from build123d import *

# Parameters (mm, degrees)
BOSS_EXTRUDE1_DEPTH       = 10
SKETCH3_W                 = 6
SKETCH3_H                 = 5
CHAMFER1_SIZE             = 4
SKETCH10_R                = 6.5
CUT_EXTRUDE1_DEPTH        = 11
F_6_0MM_DOWEL_HOLE1_D     = 6
F_6_0MM_DOWEL_HOLE1_DEPTH = 4
F_6_0MM_DOWEL_HOLE1_TIP   = 1.802581857


with BuildPart() as part:
    # Sketch1 → Boss-Extrude1 (new body)
    with BuildSketch(Plane(origin=(0, 0, 0), x_dir=(1, 0, 0), z_dir=(0, 1, 0))):
        Polygon((0, -85), (0, -50), (-50, -50), (-50, 50), (0, 50), (0, 85), (-85, 85), (-85, -85), align=None)
    extrude(amount=BOSS_EXTRUDE1_DEPTH)

    # Cut-Sweep1: sweep along a path in Sketch4
    with BuildLine(Plane.XZ) as cut_sweep1_path:
        Line((0, 50), (-50, 50))
        Line((-50, 50), (-50, -50))
        Line((-50, -50), (0, -50))
    # Sketch3 → Cut-Sweep1 (sweep, cut)
    with BuildSketch(Plane(origin=(0, 0, 0), x_dir=(0, 0, -1), z_dir=(1, 0, 0))):
        with Locations((-53, 2.5)):
            Rectangle(SKETCH3_W, SKETCH3_H)
    sweep(path=cut_sweep1_path.line, transition=Transition.RIGHT, mode=Mode.SUBTRACT)

    # Chamfer1
    chamfer1_edges = [part.edges().sort_by_distance(p)[0] for p in [
        (0, 10, 67.5),
        (0, 10, -67.5),
    ]]
    chamfer(chamfer1_edges, length=CHAMFER1_SIZE)

    # Sketch10 → Cut-Extrude1 (cut, through all)
    with BuildSketch(Plane(origin=(0, 10, 0), x_dir=(1, 0, 0), z_dir=(0, 1, 0))):
        with Locations((-72.499960031, 0)):
            Circle(SKETCH10_R)
        with Locations((-20, -72.5)):
            Circle(SKETCH10_R)
        with Locations((-20, 72.5)):
            Circle(SKETCH10_R)
    extrude(amount=-CUT_EXTRUDE1_DEPTH, mode=Mode.SUBTRACT)

    # 6.0mm Dowel Hole1
    with Locations(Plane(origin=(0, 10, 0), x_dir=(1, 0, 0), z_dir=(0, 1, 0))):
        with Locations((-72.5, -72.5)):
            Hole(F_6_0MM_DOWEL_HOLE1_D / 2, depth=F_6_0MM_DOWEL_HOLE1_DEPTH)
            with Locations((0, 0, -(F_6_0MM_DOWEL_HOLE1_DEPTH + F_6_0MM_DOWEL_HOLE1_TIP / 2))):  # 118° drill point
                Cone(0, F_6_0MM_DOWEL_HOLE1_D / 2, F_6_0MM_DOWEL_HOLE1_TIP, mode=Mode.SUBTRACT)

    # Cut-Sweep2: sweep along a path in Sketch5
    with BuildLine(Plane(origin=(0, 10, 0), x_dir=(1, 0, 0), z_dir=(0, 1, 0))) as cut_sweep2_path:
        Line((0, -72), (-20, -52))
        Line((-20, -52), (-52, -52))
        Line((-52, -52), (-52, 52))
        Line((-52, 52), (-20, 52))
        Line((-20, 52), (0, 72))
    # Sketch9 → Cut-Sweep2 (sweep, cut)
    with BuildSketch(Plane(origin=(36, 0, 36), x_dir=(0, -1, 0), z_dir=(0.707106781, 0, 0.707106781))):
        Polygon((-10, -50.911688245), (-10, -51.911688245), (-9, -50.911688245), (-10, -49.911688245), align=None)
    sweep(path=cut_sweep2_path.line, transition=Transition.RIGHT, mode=Mode.SUBTRACT)


solid = part.part
Can you work these out from the model? Positions are in its coordinate system, mm. A direction names the side the tool comes from. Coordinates: 2 decimals unless noted, no trailing zeros. Loops run counter-clockwise (first coordinate to the right, second up) from the corner with the lowest first, then second, coordinate; pieces in that order, holes last. Notation, with made-up numbers: M -27.75,68 L -16.75,68 A26 cw -16.75,98 Z; hole C 32.25,50.25 d2. An arc over 180 degrees is marked long. Answer as CSV lines item,"result". Start each with the question number.
1. Thinking about a two-plate mould opening in X: for faces 1 (the face through (-79, 5, 0)), 2 (the face through (-54, 10, -1)), 3 (the face through (-2, 8, 68)), 4 (the face through (-11.98, 9.51, 60.74)), which applies, +X half, -X half, draft (parallel to the pull), parting line (faces both ways), or undercut?
2. For faces 5 (the face through (-56, 3, -1)), 6 (the face through (-50, 7, 1)), 7 (the face through (-21.409, 5.07, 78.845)), 8 (the face through (-11.18, 9.49, -60.13)), which set-ups out of +Z, -Z, +X, -X, +Y, -Y let a thin tool reach every point of the face, with its end or its side?
3. Suppose I cut it at A-A, the plane z = -72.5. List the corners of the cut face in (x, y) for me.
4. Suppose I cut it at B-B, the plane y = 2.25. List the corners of the cut face in (x, z) for me, plus the area to 3 significant figures.
5. If I drill on probe 1 along Z at (x, y) = (-20, 6.75); probe 2 along Z at (x, y) = (-72.5, 8.05); probe 3 along Z at (x, y) = (-34, 8), over which ranges is the centre line in solid material (lowest first)? Write a range as [from, to].
6. Suppose I cut it at D-D, the plane z = -39. List the corners of the cut face in (x, y) for me, plus the area to 3 significant figures.
7. Suppose I cut it at C-C, the plane z = 0. List the corners of the cut face in (x, y) for me.
8. For pin 1 Ø2.5 at (y, z) = (3.5, 9.5) entering from +X; pin 2 Ø1.5 at (y, z) = (7, -14) entering from +X, each with a flat end and sliding along its axis, tell me the tip position at first contact or that it passes through.
Output:
1,face 1,"undercut"
1,face 2,"draft"
1,face 3,"+X half"
1,face 4,"undercut"
2,face 5,"+X, -Y"
2,face 6,"+X, +Y, -Y"
2,face 7,"+Y, -Y"
2,face 8,"+Y"
3,outline,"M -85,0 L -26.5,0 L -26.5,10 L -85,10 Z; M -13.5,0 L 0,0 L 0,6 L -4,10 L -13.5,10 Z"
4,outline,"M -85,-85 L 0,-85 L 0,-56 L -56,-56 L -56,56 L 0,56 L 0,85 L -85,85 Z; hole C -72.5,0 d13; hole C -20,-72.5 d13; hole C -20,72.5 d13"
4,area,"7,780 mm^2"
5,probe 1,"z = [-85, -79], [-66, -50], [50, 66], [79, 85]"
5,probe 2,"z = [-85, -6.5], [6.5, 69.5], [75.5, 85]"
5,probe 3,"z = [-85, -50], [50, 85]"
6,outline,"M -85,0 L -56,0 L -56,5 L -50,5 L -50,10 L -51,10 L -52,9 L -53,10 L -85,10 Z"
6,area,"319 mm^2"
7,outline,"M -85,0 L -79,0 L -79,10 L -85,10 Z; M -66,0 L -56,0 L -56,5 L -50,5 L -50,10 L -51,10 L -52,9 L -53,10 L -66,10 Z"
8,pin 1,"stops at x = -56"
8,pin 2,"stops at x = -50"
